Source: CAD feature listing. Evaluate the final solid. Frame: model axes, mm. Face numbers are marked on the shaded views. Round coordinates to 2 decimals unless told otherwise and drop trailing zeros. Order: outer loops, then holes, each group sorted by start corner. A loop starts at its lowest first (then second) coordinate and runs counter-clockwise, first axis right, second up.
```python
from build123d import *

# Parameters (mm, degrees)
SKETCH_1_R          = 12
EXTRUDE_522_DEPTH   = 22.3
SKETCH_2_OUTSIDE_W  = 336.56
SKETCH_2_OUTSIDE_H  = 331.262
SKETCH_2_OUTSIDE_R  = 17.12565236
CUT_EXTRUDE_1_DEPTH = 38
CUT_EXTRUDE_1_DRAFT = -75
SKETCH_3_OUTSIDE_W  = 336.56
SKETCH_3_OUTSIDE_H  = 331.262
SKETCH_3_OUTSIDE_R  = 17.12565236
CUT_EXTRUDE_2_DEPTH = 38
CUT_EXTRUDE_2_DRAFT = -75
CHAMFER_1_SIZE      = 0.2


with BuildPart() as part:
    # 草图1 → Extrude 522 (new body)
    with BuildSketch(Plane.XY):
        Polygon((9.8875, 17.12565236), (-9.8875, 17.12565236), (-19.775, 0), (-9.8875, -17.12565236), (9.8875, -17.12565236), (19.775, 0), align=None)
        Circle(SKETCH_1_R, mode=Mode.SUBTRACT)
    extrude(amount=EXTRUDE_522_DEPTH)


with BuildPart() as cut_extrude_1_tool:
    # 草图2 outside → 切除-拉伸1 (with draft: the straight prism first)
    with BuildSketch(Plane(origin=(0, 0, 0), x_dir=(-1, 0, 0), z_dir=(0, 0, -1))):
        Rectangle(SKETCH_2_OUTSIDE_W, SKETCH_2_OUTSIDE_H)
        Circle(SKETCH_2_OUTSIDE_R, mode=Mode.SUBTRACT)
    extrude(amount=-CUT_EXTRUDE_1_DEPTH)
    # 切除-拉伸1: the draft: its side faces are tilted about the plane it starts from
    cut_extrude_1_sides = [cut_extrude_1_tool.faces().sort_by_distance(p)[0] for p in [
        (0, -165.631, 19),
        (-168.28, 0, 19),
        (0, 165.631, 19),
        (168.28, 0, 19),
        (17.12565236, 0, 19),
    ]]
    draft(cut_extrude_1_sides, Plane(origin=(0, 0, 0), x_dir=(-1, 0, 0), z_dir=(0, 0, -1)), CUT_EXTRUDE_1_DRAFT)


with BuildPart() as part_1:
    add(part.part)

    # 切除-拉伸1: cut by cut_extrude_1_tool
    add(cut_extrude_1_tool.part, mode=Mode.SUBTRACT)


with BuildPart() as cut_extrude_2_tool:
    # 草图3 outside → 切除-拉伸2 (with draft: the straight prism first)
    with BuildSketch(Plane.XY.offset(22.3)):
        Rectangle(SKETCH_3_OUTSIDE_W, SKETCH_3_OUTSIDE_H)
        Circle(SKETCH_3_OUTSIDE_R, mode=Mode.SUBTRACT)
    extrude(amount=-CUT_EXTRUDE_2_DEPTH)
    # 切除-拉伸2: the draft: its side faces are tilted about the plane it starts from
    cut_extrude_2_sides = [cut_extrude_2_tool.faces().sort_by_distance(p)[0] for p in [
        (0, -165.631, 3.3),
        (168.28, 0, 3.3),
        (0, 165.631, 3.3),
        (-168.28, 0, 3.3),
        (-17.12565236, 0, 3.3),
    ]]
    draft(cut_extrude_2_sides, Plane.XY.offset(22.3), CUT_EXTRUDE_2_DRAFT)


with BuildPart() as part_2:
    add(part_1.part)

    # 切除-拉伸2: cut by cut_extrude_2_tool
    add(cut_extrude_2_tool.part, mode=Mode.SUBTRACT)

    # 倒角1
    chamfer_1_edges = [part_2.edges().sort_by_distance(p)[0] for p in [
        (-12, 0, 0),
        (-12, 0, 22.3),
    ]]
    chamfer(chamfer_1_edges, length=CHAMFER_1_SIZE)


solid = part_2.part
```
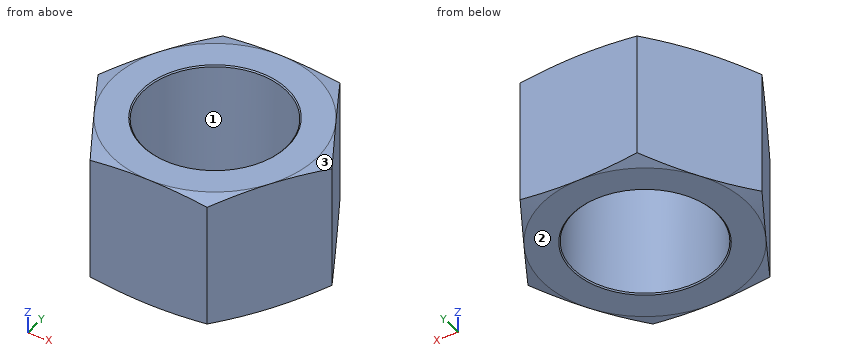
1. Section A-A on z = 7.25. Return loops of the section in (x, y) (1 decimal), plus the area to 3 significant figures.
2. First-contact query: pin 1 (6 mm diameter, centred on x = -14, z = 14, fed in from +Y); pin 2 (1.5 mm diameter, centred on x = -14.5, z = 17, fed in from +Y); pin 3 (2 mm diameter, centred on y = -4.5, z = 5.5, fed in from +X). Flat tips, straight axial feed; report the tip coordinate or a pass-through.
3. Pull-direction query (Z, two-part tool) for the marked faces 1, 2 and 3; classes: released by +Z, released by -Z, zero draft, split by the parting line, or undercut.
4. Line query: line 1 along Y through (x, z) = (0, 5); line 2 along X through (y, z) = (4, 19.5); line 3 along X through (y, z) = (8, 12.75). Output: solid intervals per line, ascending.
Result:
1. outline: (-19.8, 0) - (-9.9, -17.1) - (9.9, -17.1) - (19.8, 0) - (9.9, 17.1) - (-9.9, 17.1) - close; hole circle Ø24 at (0, 0)
1. area: 564 mm2
2. pin 1: stops at y = 15.2
2. pin 2: stops at y = 10.44
2. pin 3: stops at x = 17.75
3. face 1: zero draft
3. face 2: released by -Z
3. face 3: released by +Z
4. line 1: y = -17.13 to -12, 12 to 17.13
4. line 2: x = -17.47 to -11.31, 11.31 to 17.47
4. line 3: x = -15.16 to -8.94, 8.94 to 15.16
